```python
from build123d import *

# Parameters (mm, degrees)
BOSS_EXTRUDE1_DEPTH = 10


with BuildPart() as part:
    # Sketch1 → Boss-Extrude1 (new body)
    with BuildSketch(Plane(origin=(0, 0, 0), x_dir=(1, 0, 0), z_dir=(0, 1, 0))):
        Polygon((2.886751346, 0), (1.443375673, 2.5), (-1.443375673, 2.5), (-2.886751346, 0), (-1.443375673, -2.5), (1.443375673, -2.5), align=None)
    extrude(amount=BOSS_EXTRUDE1_DEPTH)

    # Sketch3 → Cut-Revolve1 (revolve, cut)
    with BuildSketch(Plane.XY, mode=Mode.PRIVATE) as cut_revolve1_sk:
        with BuildLine():
            Line((-2, 10), (-2, 10.901570298))
            Line((-2, 10.901570298), (-4.378417403, 10.901570298))
            Line((-4.378417403, 10.901570298), (-4.378417403, 5))
            Line((-4.378417403, 5), (-2.886751346, 5))
            ThreePointArc((-2.886751346, 5), (-2.607836376, 5.276622353), (-2.266701974, 5.471406351))
            ThreePointArc((-2.266701974, 5.471406351), (-1.950264944, 5.90495326), (-2, 6.439389168))
            ThreePointArc((-2, 6.439389168), (-2.964233791, 8.219694584), (-2, 10))
        make_face()
    revolve(cut_revolve1_sk.sketch.rotate(Axis((0, -0.795078515, 0), (0, 1, 0)), 270), axis=Axis((0, -0.795078515, 0), (0, 1, 0)), mode=Mode.SUBTRACT)


solid = part.part
```
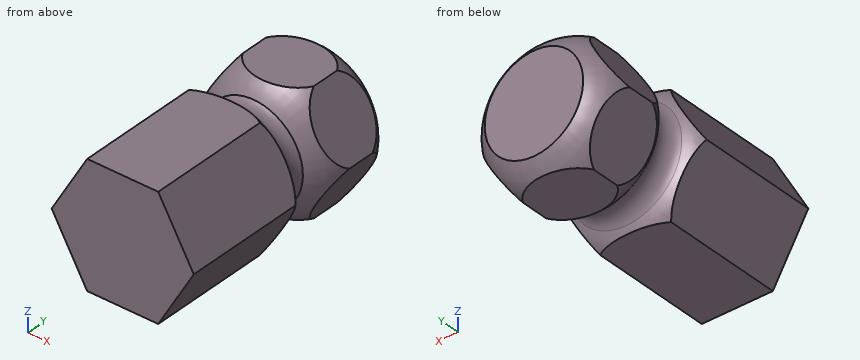
CAD build for the part. Positions are in the model's coordinates, mm. Give positions to 0.01 mm unless a question says otherwise; leave off trailing zeros. Write each loop counter-clockwise with the first axis right and the second up, starting at its lowest first coordinate (ties: lowest second). Pieces come first, ordered by that corner, then holes. Notation, with made-up numbers: (57.5, 86) -> (115.5, 86) arc R16 cw to (115.5, 92) -> close; hole circle Ø3 at (6.25, 22.5). An arc over 180 degrees is marked (long way). Write each question's results on one line, items separated by ' | '.
1. Cut at B-B, the plane y = 6.25. Write the cut outline in (x, z).
Geometry check:
outline: circle Ø3.87 at (0, 0)
2. Cut at A-A, the plane y = 4. Write the cut outline in (x, z), then the cut area to 3 significant figures.
Geometry check:
outline: (-2.89, 0) -> (-1.44, -2.5) -> (1.44, -2.5) -> (2.89, 0) -> (1.44, 2.5) -> (-1.44, 2.5) -> close | area: 21.7 mm²
3. Wall check: probe 1 along Y at (x, z) = (-1.5, -1.5); probe 2 along Y at (x, z) = (-2.2, -0.2); probe 3 along X at (y, z) = (8.75, 0.5). Give the ranges that are in metal, low to high. Write a range as [from, to].
Geometry check:
probe 1: [0, 5.6], [6.52, 9.91] | probe 2: [0, 5.51], [6.59, 9.84] | probe 3: [-2.6, 2.6]
